Design review of the part built by this model. Coordinates are the model's own, in mm. Face numbers are marked on the shaded views. A direction names the side the tool comes from. Give positions to 0.01 mm unless a question says otherwise; leave off trailing zeros. Loops run counter-clockwise (first coordinate to the right, second up) from the corner with the lowest first, then second, coordinate; pieces in that order, holes last.
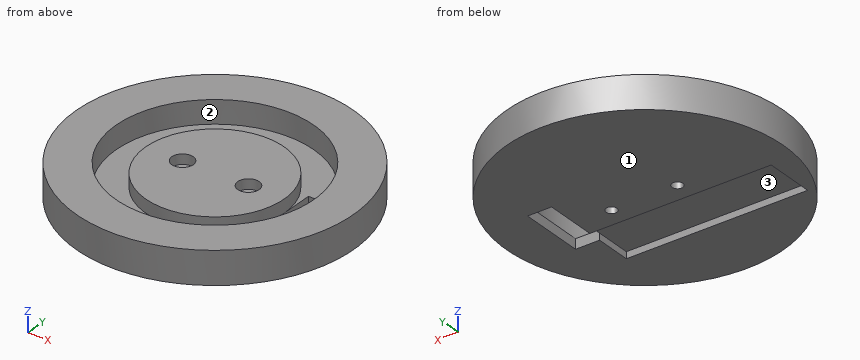
from build123d import *

# Parameters (mm, degrees)
F2_W           = 7.2961132542
F2_H           = 9.9664424297
F2_H_2         = 9.7550563514
F3_DEPTH       = 25
F4_W           = 55
F4_H           = 15
F5_DEPTH       = 2
F7_D           = 3.3
F7_CBORE_D     = 6.5
F7_CBORE_DEPTH = 3


with BuildPart() as f1:
    # F0 (on Front) → F1 (revolve)
    with BuildSketch(Plane.XZ):
        Polygon((-42, 0), (0, 0), (0, 7), (-21, 7), (-21, 3), (-30, 3), (-30, 10), (-42, 10), align=None)
    revolve(axis=Axis((0, 0, 3.5), (0, 0, 1)))

    # F2 (on face) → F3 (cut)
    with BuildSketch(Plane.XY.offset(3)):
        with Locations((24.6480566271, 4.9832212149)):
            Rectangle(F2_W, F2_H)
        with Locations((24.6480566271, -4.8775281757)):
            Rectangle(F2_W, F2_H_2)
    extrude(amount=-F3_DEPTH, mode=Mode.SUBTRACT)

    # F4 (on face) → F5 (cut)
    with BuildSketch(Plane(origin=(0, 0, 0), x_dir=(1, 0, 0), z_dir=(0, 0, -1))):
        with Locations((-6.5, 13.2730269618)):
            Rectangle(F4_W, F4_H)
    extrude(amount=-F5_DEPTH, mode=Mode.SUBTRACT)

    # F7 (through all)
    with Locations(Plane.XY.offset(7)):
        with Locations((-9.8275868147, 0), (10.1724131853, 0)):
            CounterBoreHole(F7_D / 2, F7_CBORE_D / 2, F7_CBORE_DEPTH)


solid = f1.part
Q1. Take a section at D-D (y = -24.5). Give the boundary of the cut face in (x, z), plus the area to 3 significant figures.
Results:
outline: (-34.11, 0) - (34.11, 0) - (34.11, 10) - (17.31, 10) - (17.31, 3) - (-17.31, 3) - (-17.31, 10) - (-34.11, 10) - close
area: 440 mm2
Q2. Take a section at A-A (x = 0). Give the boundary of the cut face in (y, z), plus the area to 3 significant figures.
Results:
outline: (-42, 0) - (-20.77, 0) - (-20.77, 2) - (-5.77, 2) - (-5.77, 0) - (42, 0) - (42, 10) - (30, 10) - (30, 3) - (21, 3) - (21, 7) - (-21, 7) - (-21, 3) - (-30, 3) - (-30, 10) - (-42, 10) - close
area: 558 mm2
Q3. Insertion check: pin 1 (7.5 mm diameter, centred on x = 10.17, y = 0, fed in from +Z); pin 2 (1.5 mm diameter, centred on x = 25, z = 1.5, fed in from +Y); pin 3 (7.5 mm diameter, centred on x = -15, y = -16, fed in from -Z). Each pin has a flat end and moves straight along its axis. Give the tip position at first contact, or say it passes through.
Results:
pin 1: stops at z = 7
pin 2: stops at y = 34.29
pin 3: stops at z = 2
Q4. Wall thickness on line 1 (Y direction, x = 16, z = 4); line 2 (X direction, y = -12, z = 5.5); line 3 (X direction, y = -4, z = 6.75): over which ranges is each line inside the solid? List them lowest first.
Results:
line 1: y = -38.83 to -25.38, -13.6 to 13.6, 25.38 to 38.83
line 2: x = -40.25 to -27.5, -17.23 to 17.23, 27.5 to 40.25
line 3: x = -41.81 to -29.73, -20.62 to 20.62, 29.73 to 41.81
Q5. Tool access review of the marked faces 1, 2 and 3: name each direction out of +Z, -Z, +X, -X, +Y, -Y from which nothing blocks a thin tool from reaching the whole face with its end or side.
Results:
face 1: -Z, +X, -X, +Y, -Y
face 2: +Z
face 3: -Z
Q6. Take a section at B-B (y = -8). Give the boundary of the cut face in (x, z), plus the area to 3 significant figures.
Results:
outline: (-41.23, 0) - (-34, 0) - (-34, 2) - (21, 2) - (21, 3) - (19.42, 3) - (19.42, 7) - (-19.42, 7) - (-19.42, 3) - (-28.91, 3) - (-28.91, 10) - (-41.23, 10) - close; (28.3, 0) - (41.23, 0) - (41.23, 10) - (28.91, 10) - (28.91, 3) - (28.3, 3) - close
area: 443 mm2
Q7. Take a section at C-C (x = 24.5). Give the boundary of the cut face in (y, z), plus the area to 3 significant figures.
Results:
outline: (-34.11, 0) - (-9.76, 0) - (-9.76, 3) - (-17.31, 3) - (-17.31, 10) - (-34.11, 10) - close; (9.97, 0) - (34.11, 0) - (34.11, 10) - (17.31, 10) - (17.31, 3) - (9.97, 3) - close
area: 381 mm2
